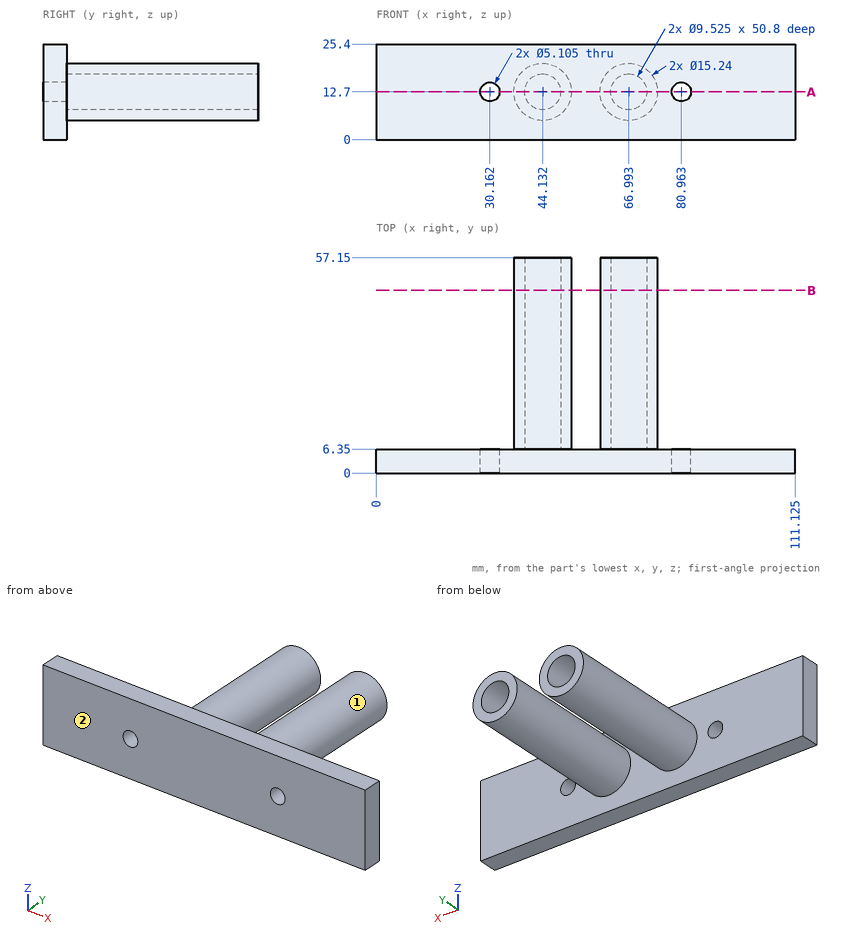
Here's the drawing with two shaded views (mm, measured from the low corner). I have some questions. Round coordinates to 2 decimals unless told otherwise and drop trailing zeros. Write each loop counter-clockwise with the first axis right and the second up, starting at its lowest first coordinate (ties: lowest second). Pieces come first, ordered by that corner, then holes. Notation, with made-up numbers: M 36,25.5 L 84,25.5 A19 cw 84,38.5 Z; hole C 35,25 d2. An arc over 180 degrees is marked long. Answer in a Markdown table with one row per item. Add a question column.
Q1. Imagine slicing it at A-A (z = 12.7). Give the number of separate pieces and of enclosed holes in the cut face, then the cut area to 3 significant figures.
Q2. Will these pins go through, and if not, where does the flat tip stop? pin 1 Ø6 at (x, y) = (48.5, 45.5) entering from -Z; pin 2 Ø3 at (x, z) = (45.5, 13) entering from +Y.
Q3. Imagine slicing it at B-B (y = 48.5). Please give me the cut outline in (x, z) (1 decimal), then the cut area to 3 significant figures.
Q4. If I drill on line 1 (X direction, y = 4, z = 12.7) (1 decimal); line 2 (X direction, y = 34.5, z = 12.7) (1 decimal); line 3 (X direction, y = 30.5, z = 12.25) (1 decimal), over which ranges is the centre line in solid material (lowest first)? Write a range as from..to.
Q5. If we mould it in two halves opening along X, with no side actions, what happens to the marked faces 1 and 2? For each: +X half, -X half, draft (parallel to the pull), parting line (faces both ways), or undercut.
Values:
| question | item | result |
|---|---|---|
| 1 | separate pieces | 3 |
| 1 | enclosed holes | 0 |
| 1 | area | 1,220 mm^2 |
| 2 | pin 1 | z = 5.2 |
| 2 | pin 2 | y = 6.35 |
| 3 | outline | C 44.1,12.7 d15.2; C 67,12.7 d15.2; hole C 44.1,12.7 d9.5; hole C 67,12.7 d9.5 |
| 3 | area | 222 mm^2 |
| 4 | line 1 | 0..27.6, 32.7..78.4, 83.5..111.1 |
| 4 | line 2 | 36.5..39.4, 48.9..51.8, 59.4..62.2, 71.8..74.6 |
| 4 | line 3 | 36.5..39.4, 48.9..51.7, 59.4..62.3, 71.7..74.6 |
| 5 | face 1 | undercut |
| 5 | face 2 | draft |
